Input: part model. Units: mm. Frame: model coordinates. Face numbers are marked on the shaded views. A direction names the side the tool comes from. Coordinates: 2 decimals unless noted, no trailing zeros. Loops run counter-clockwise (first coordinate to the right, second up) from the corner with the lowest first, then second, coordinate; pieces in that order, holes last. Notation, with made-up numbers: (-15.75, 56.25) - (-2.75, 56.25) arc R4 cw to (-2.75, 60.25) - close; hole circle Ø3 at (89.5, -1.5). An arc over 180 degrees is marked (long way). Use a Markdown table: item, result. Add a question column.
1. Draft query along Z for the marked faces 3, 4 and 5. Return one class per face: released by +Z, released by -Z, zero draft, split by the parting line, or undercut.
2. Section query B-B on z = 4. Return the cut outline in (x, y), then the cut area to 3 significant figures.
3. Contact query for flat-ended pins moving along their axis: P1, Ø8, axis at y = 11.5, z = 8, coming from the +X side; P2, Ø6, axis at y = 3.5, z = 18.5, coming from the -X side; P3, Ø3, axis at x = -11, z = 7.5, coming from the +Y side; P4, Ø6, axis at x = 5.5, y = 6.5, coming from the -Z side. Output: stop coordinate, or through.
4. Ray query, L1, parallel to Z at x = -8.5, y = 7; L2, parallel to Z at x = -4, y = -13; L3, parallel to Y at x = -0.5, z = 22. Return the intervals inside material, ascending. Write a range as [from, to].
5. Section query A-A on z = 20. Return the cut outline in (x, y).
6. Access query for the marked faces 1 and 2. Directions: +Z, -Z, +X, -X, +Y, -Y. A direction counts if a zero-diameter tool reaches every point of the face in a straight line with its end or side. Return the directions, or none.
```python
from build123d import *

# Parameters (mm, degrees)
F0_R      = 19.0458801966
F2_DEPTH  = 5.08
F1_R      = 16.5564413769
F3_DEPTH  = 15.24
F5_R      = 10.7565912882
F6_DEPTH  = 25.4
F7_R      = 15.4966869389
F8_DEPTH  = 2.54
F9_R      = 13.1720463189
F10_DEPTH = 2.54
F11_R     = 10.9761291002
F12_DEPTH = 2.54
F13_R     = 13.5071591259
F14_DEPTH = 1.27
F15_R     = 13.5553537987
F16_DEPTH = 12.7


# Not quite as in the source:
# - a fillet or chamfer that OpenCascade refuses, or shapes differently, is made with other operations: its cross-section is extruded or revolved along the edge and cut away or added


with BuildPart() as f2:
    # F0 (on Top) → F2 (new body)
    with BuildSketch(Plane.XY):
        Circle(F0_R)
    extrude(amount=F2_DEPTH)

    # F1 (on Top) → F3 (join)
    with BuildSketch(Plane.XY):
        Circle(F1_R)
    extrude(amount=F3_DEPTH)

    # F4: fillet of radius 12.7 on 1 edges, made by hand

    # F4_s1 → F4_t2 (revolve, cut)
    with BuildSketch(Plane.XZ):
        with BuildLine():
            ThreePointArc((16.5564413769, 5.08), (12.1452187403, 12.3773776994), (4.1130334835, 15.24))
            Line((4.1130334835, 15.24), (16.5564413769, 15.24))
            Line((16.5564413769, 15.24), (16.5564413769, 5.08))
        make_face()
    revolve(axis=Axis((0, 0, 15.24), (0, 0, 1)), mode=Mode.SUBTRACT)

    # F5 (on Top) → F6 (join)
    with BuildSketch(Plane.XY):
        Circle(F5_R)
    extrude(amount=F6_DEPTH)

    # F7 (on face) → F8 (join)
    with BuildSketch(Plane.XY.offset(25.4)):
        Circle(F7_R)
    extrude(amount=F8_DEPTH)

    # F9 (on face) → F10 (join)
    with BuildSketch(Plane.XY.offset(27.94)):
        Circle(F9_R)
    extrude(amount=F10_DEPTH)

    # F11 (on face) → F12 (join)
    with BuildSketch(Plane.XY.offset(30.48)):
        Circle(F11_R)
    extrude(amount=F12_DEPTH)

    # F13 (on face) → F14 (join)
    with BuildSketch(Plane.XY.offset(33.02)):
        Circle(F13_R)
    extrude(amount=F14_DEPTH)

    # F15 (on face) → F16 (join)
    with BuildSketch(Plane.XY.offset(34.29)):
        Circle(F15_R)
    extrude(amount=F16_DEPTH)


solid = f2.part
```
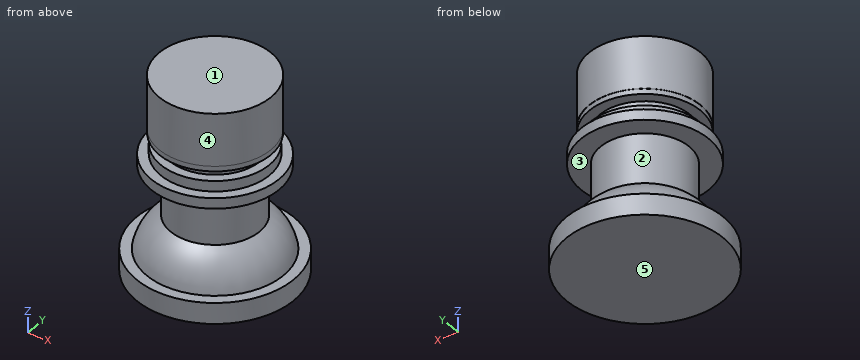
Resolved:
| question | item | result |
|---|---|---|
| 1 | face 3 | undercut |
| 1 | face 4 | zero draft |
| 1 | face 5 | released by -Z |
| 2 | outline | circle Ø38.09 at (0, 0) |
| 2 | area | 1,140 mm² |
| 3 | P1 | x = 16.91 |
| 3 | P2 | x = -10.74 |
| 3 | P3 | y = 12.84 |
| 3 | P4 | z = 0 |
| 4 | L1 | [0, 13.2], [25.4, 30.48], [33.02, 46.99] |
| 4 | L2 | [0, 10.98], [25.4, 27.94] |
| 4 | L3 | [-10.74, 10.74] |
| 5 | outline | circle Ø21.51 at (0, 0) |
| 6 | face 1 | +Z, +X, -X, +Y, -Y |
| 6 | face 2 | none |
